The drawing under review shows one solid part. Ordinate dimensions are in mm from its lowest x, y, z. A direction names the side the tool comes from. Round coordinates to 2 decimals unless told otherwise and drop trailing zeros. Loops run counter-clockwise (first coordinate to the right, second up) from the corner with the lowest first, then second, coordinate; pieces in that order, holes last. Notation, with made-up numbers: (42, -1.5) -> (57, -1.5) arc R20 cw to (57, 32.5) -> close; hole circle Ø2 at (-23, 32). An arc over 180 degrees is marked (long way). Use a Markdown table: item, result. Add a question column.
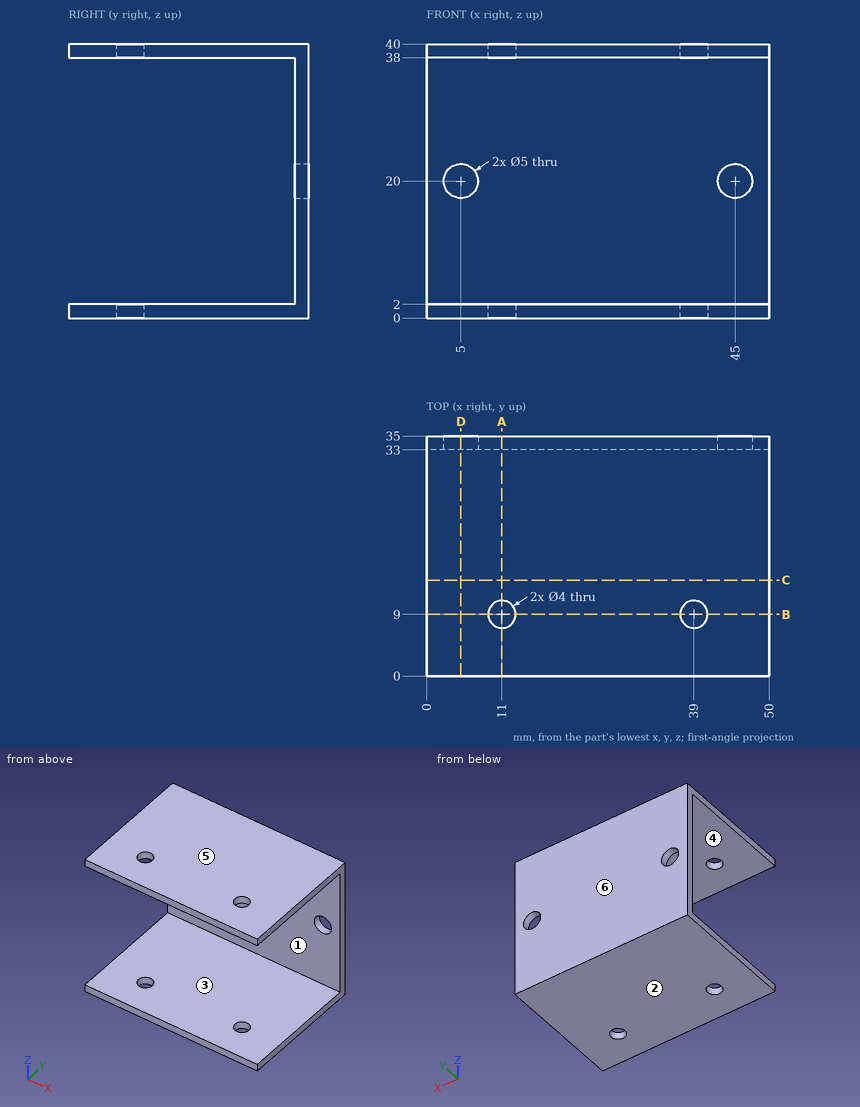
1. Consider section B-B on y = 9. State the section outline as (x, z) points.
2. To check wall thickness, follow probe 1 along X at (y, z) = (34.05, 20); probe 2 along Y at (x, z) = (39, 39.6); probe 3 along Z at (x, y) = (4, 25). State the ranges of each line that lie inside material, in increasing order. Write a range as from..to.
3. Consider section A-A on x = 11. State the section outline as (y, z) points, plus the area to 3 significant figures.
4. Mouldability with a two-part tool opening along Z and no side actions: class the marked faces 3, 4, 5 and 6 as +Z half, -Z half, draft (parallel to the pull), parting line (faces both ways), or undercut.
5. Consider section C-C on y = 14. State the section outline as (x, z) points.
6. Consider section D-D on x = 5. State the section outline as (y, z) points, plus the area to 3 significant figures.
7. For the marked faces 1 and 2, list the 3-axis set-ups (+Z, -Z, +X, -X, +Y, -Y) from which the entire face can be reached by the end or side of a thin tool; tool diameter is ignored.
8. Insertion check: P1, Ø6, axis at x = 5, z = 20, coming from the -Y side. The pin has a flat end and moves straight along its axis. Give the tip position at first contact, or say it passes through.
Verdict:
| question | item | result |
|---|---|---|
| 1 | outline | (0, 0) -> (9, 0) -> (9, 2) -> (0, 2) -> close; (0, 38) -> (9, 38) -> (9, 40) -> (0, 40) -> close; (13, 0) -> (37, 0) -> (37, 2) -> (13, 2) -> close; (13, 38) -> (37, 38) -> (37, 40) -> (13, 40) -> close; (41, 0) -> (50, 0) -> (50, 2) -> (41, 2) -> close; (41, 38) -> (50, 38) -> (50, 40) -> (41, 40) -> close |
| 2 | probe 1 | x = 0..2.5, 7.5..42.5, 47.5..50 |
| 2 | probe 2 | y = 0..7, 11..35 |
| 2 | probe 3 | z = 0..2, 38..40 |
| 3 | outline | (0, 0) -> (7, 0) -> (7, 2) -> (0, 2) -> close; (0, 38) -> (7, 38) -> (7, 40) -> (0, 40) -> close; (11, 0) -> (35, 0) -> (35, 40) -> (11, 40) -> (11, 38) -> (33, 38) -> (33, 2) -> (11, 2) -> close |
| 3 | area | 196 mm² |
| 4 | face 3 | undercut |
| 4 | face 4 | undercut |
| 4 | face 5 | +Z half |
| 4 | face 6 | draft |
| 5 | outline | (0, 0) -> (50, 0) -> (50, 2) -> (0, 2) -> close; (0, 38) -> (50, 38) -> (50, 40) -> (0, 40) -> close |
| 6 | outline | (0, 0) -> (35, 0) -> (35, 17.5) -> (33, 17.5) -> (33, 2) -> (0, 2) -> close; (0, 38) -> (33, 38) -> (33, 22.5) -> (35, 22.5) -> (35, 40) -> (0, 40) -> close |
| 6 | area | 202 mm² |
| 7 | face 1 | +X, -X, -Y |
| 7 | face 2 | -Z, +X, -X, +Y, -Y |
| 8 | P1 | stops at y = 33 |
